```python
from build123d import *

# Parameters (mm, degrees)
BOSS_EXTRUDE1_DEPTH = 4.7625
CUT_EXTRUDE5_DEPTH  = 591.371112999
SCALE1_SCALE_X      = 0.622
SCALE1_SCALE_Y      = 0.625
SCALE1_SCALE_Z      = 1
CUT_EXTRUDE8_DEPTH  = 422.073439333
FILLET1_R           = 10.16
CUT_EXTRUDE9_DEPTH  = 422.073439333
BOSS_EXTRUDE2_DEPTH = 4.7625
CUT_EXTRUDE10_DEPTH = 422.073439333
CUT_EXTRUDE11_DEPTH = 422.073439333
SKETCH16_W          = 50.8
SKETCH16_H          = 6.35
BOSS_EXTRUDE3_DEPTH = 4.7625
CUT_EXTRUDE12_START = -4.7625
CUT_EXTRUDE12_DEPTH = 4.7625
CUT_EXTRUDE13_DEPTH = 421.232758824


# Read off the part's stored shape, not the designer's step: Cut-Extrude12
with BuildPart() as part:
    # Sketch3 → Boss-Extrude1 (new body)
    with BuildSketch(Plane.XY):
        Polygon((312.000738686, 65.991135768), (166.792028218, 317.5), (-166.792028218, 317.5), (-312.000738686, 65.991135768), (-276.650369343, 4.7625), (276.650369343, 4.7625), align=None)
        Polygon((-166.792028218, 317.5), (166.792028218, 317.5), (60.750369343, 501.169540891), (-60.750369343, 501.169540891), align=None)
    extrude(amount=BOSS_EXTRUDE1_DEPTH)

    # Sketch7 → Cut-Extrude5 (cut, through all)
    with BuildSketch(Plane.XY.offset(4.7625)):
        with BuildLine():
            Line((-147.068010972, 237.363), (147.068010972, 237.363))
            ThreePointArc((147.068010972, 237.363), (158.0665336, 243.713), (158.0665336, 256.413))
            Line((158.0665336, 256.413), (49.751846715, 444.019540891))
            ThreePointArc((49.751846715, 444.019540891), (45.103324087, 448.668063519), (38.753324087, 450.369540891))
            Line((38.753324087, 450.369540891), (-38.753324087, 450.369540891))
            ThreePointArc((-38.753324087, 450.369540891), (-45.103324087, 448.668063519), (-49.751846715, 444.019540891))
            Line((-49.751846715, 444.019540891), (-158.0665336, 256.413))
            ThreePointArc((-158.0665336, 256.413), (-158.0665336, 243.713), (-147.068010972, 237.363))
        make_face()
    extrude(amount=-CUT_EXTRUDE5_DEPTH, mode=Mode.SUBTRACT)


with BuildPart() as part_1:
    # Scale1: scaled about (0, 161.134641619, 2.38125)
    add(part.part.scale((SCALE1_SCALE_X, SCALE1_SCALE_Y, SCALE1_SCALE_Z), about=(0, 161.134641619, 2.38125)))

    # Sketch11 → Cut-Extrude8 (cut, through all)
    with BuildSketch(Plane.XY.offset(4.7625)):
        Polygon((25.4, 183.377365607), (25.4, 88.802053107), (172.163821071, 88.802053107), (117.822833735, 183.377365607), align=None)
        Polygon((-117.822833735, 183.377365607), (-25.4, 183.377365607), (-25.4, 88.802053107), (-172.163821071, 88.802053107), align=None)
    extrude(amount=-CUT_EXTRUDE8_DEPTH, mode=Mode.SUBTRACT)

    # Fillet1
    fillet1_edges = [part_1.edges().sort_by_distance(p)[0] for p in [
        (-172.163821071, 88.802053107, 2.38125),
        (-117.822833735, 183.377365607, 2.38125),
        (-25.4, 183.377365607, 2.38125),
        (-25.4, 88.802053107, 2.38125),
        (117.822833735, 183.377365607, 2.38125),
        (172.163821071, 88.802053107, 2.38125),
        (25.4, 88.802053107, 2.38125),
        (25.4, 183.377365607, 2.38125),
    ]]
    fillet(fillet1_edges, radius=FILLET1_R)

    # Sketch12 → Cut-Extrude9 (cut, through all)
    with BuildSketch(Plane.XY.offset(4.7625)):
        Polygon((141.549539127, 193.067167281), (156.734576332, 166.639056393), (153.981648115, 165.057281684), (138.796610909, 191.485392572), align=None)
        Polygon((101.309190532, 263.101661132), (98.556262314, 261.519886423), (127.660916958, 210.866007222), (130.413845176, 212.447781931), align=None)
        Polygon((-153.981648115, 165.057281684), (-138.796610909, 191.485392572), (-141.549539127, 193.067167281), (-156.734576332, 166.639056393), align=None)
        Polygon((-127.660916958, 210.866007222), (-130.413845176, 212.447781931), (-101.309190532, 263.101661132), (-98.556262314, 261.519886423), align=None)
    extrude(amount=-CUT_EXTRUDE9_DEPTH, mode=Mode.SUBTRACT)

    # Sketch13 → Boss-Extrude2 (add)
    with BuildSketch(Plane.XY.offset(4.7625)):
        Polygon((130.413845176, 212.447781931), (141.549539127, 193.067167281), (148.526307077, 197.075871548), (137.390613126, 216.456486199), align=None)
        Polygon((-148.526307077, 197.075871548), (-137.390613126, 216.456486199), (-130.413845176, 212.447781931), (-141.549539127, 193.067167281), align=None)
    extrude(amount=-BOSS_EXTRUDE2_DEPTH)

    # Sketch14 → Cut-Extrude10 (cut, through all)
    with BuildSketch(Plane.XY.offset(4.7625)):
        Polygon((172.076529731, 63.402053107), (173.900818018, 66.577053107), (121.276529731, 66.577053107), (121.276529731, 63.402053107), align=None)
        Polygon((-121.276529731, 66.577053107), (-121.276529731, 63.402053107), (-172.076529731, 63.402053107), (-173.900818018, 66.577053107), align=None)
    extrude(amount=-CUT_EXTRUDE10_DEPTH, mode=Mode.SUBTRACT)

    # Sketch15 → Cut-Extrude11 (cut, through all)
    with BuildSketch(Plane.XY.offset(4.7625)):
        Polygon((194.064459463, 101.669950462), (192.233568098, 104.85644249), (184.98443241, 92.240012302), (187.737360627, 90.658237593), align=None)
        Polygon((173.900818018, 66.577053107), (180.227916854, 77.588765977), (177.474988636, 79.170540686), (170.239035289, 66.577053107), align=None)
        Polygon((-177.474988636, 79.170540686), (-170.239035289, 66.577053107), (-173.900818018, 66.577053107), (-180.227916854, 77.588765977), align=None)
        Polygon((-187.737360627, 90.658237593), (-184.98443241, 92.240012302), (-192.233568098, 104.85644249), (-194.064459463, 101.669950462), align=None)
    extrude(amount=-CUT_EXTRUDE11_DEPTH, mode=Mode.SUBTRACT)

    # Sketch16 → Boss-Extrude3 (add)
    with BuildSketch(Plane.XY.offset(4.7625)):
        with Locations((0, 208.777365607)):
            Rectangle(SKETCH16_W, SKETCH16_H)
    extrude(amount=-BOSS_EXTRUDE3_DEPTH)

    # Cut-Extrude12 outline → Cut-Extrude12 (cut)
    with BuildSketch(Plane.XY.offset(4.7625).offset(CUT_EXTRUDE12_START)):
        Polygon((-160.03407886, 73.810353985), (-169.67848003, 77.005839249), (-172.075093978, 69.772538371), (-170.239035289, 66.577053107), (-162.430692808, 66.577053107), align=None)
    cut_extrude12 = extrude(amount=CUT_EXTRUDE12_DEPTH, mode=Mode.SUBTRACT)

    # Mirror1: Cut-Extrude12 across plane
    add(cut_extrude12.mirror(Plane(origin=(0, 0, 0), x_dir=(0, 0, 1), z_dir=(1, 0, 0))), mode=Mode.SUBTRACT)

    # Sketch18 → Cut-Extrude13 (cut, through all)
    with BuildSketch(Plane.XY.offset(4.7625)):
        Polygon((-37.786729731, 373.656453664), (37.786729731, 373.656453664), (112.762236491, 243.168725538), (-113.438180507, 243.559444472), align=None)
    extrude(amount=-CUT_EXTRUDE13_DEPTH, mode=Mode.SUBTRACT)


solid = part_1.part
```
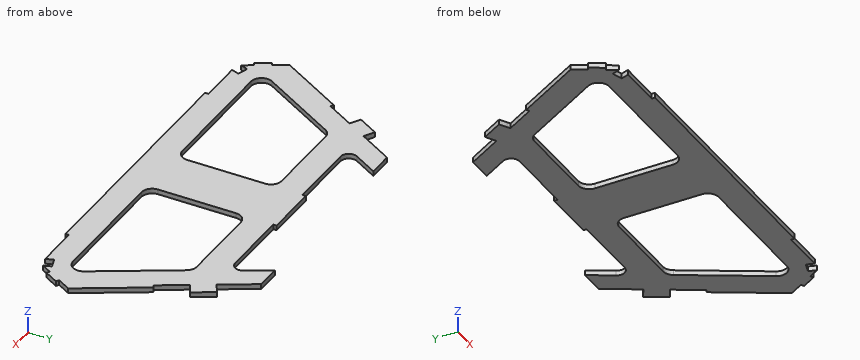
Geometry: final body of the model. Coordinates: model frame, mm. Round coordinates to 2 decimals unless told otherwise and drop trailing zeros. Order: outer loops, then holes, each group sorted by start corner. A loop starts at its lowest first (then second) coordinate and runs counter-clockwise, first axis right, second up. Notation, with made-up numbers: M -35.5,10 L -12.5,10 A18 ccw -12.5,21 Z; hole C -26.5,-16.75 d4. An arc over 180 degrees is marked long. Use one line per item in the form item = value. Start each with the question number.
Q1. Cut plane A-A (z = 1.2). Count the separate pieces of the cut face and the enclosed holes in it, and give its area (3 significant figures).
Q2. Cut plane C-C (y = 187.5). Return loops of the section in (x, z), and give its area (3 significant figures).
Q3. Pin query (flat end, axial travel): pin 1 Ø1.5 at (x, z) = (27, 1) entering from +Y; pin 2 Ø1 at (y, z) = (91, 0.5) entering from -X; pin 3 Ø2.5 at (y, z) = (144, 2.5) entering from +X. Return the tip coordinate at first contact, or that it passes through.
Q4. Material intervals for line 1 (X direction, y = 112.5, z = 3.85); line 2 (X direction, y = 214, z = 3.55); line 3 (X direction, y = 108, z = 0.6), sorted ascending. Write a range as [from, to].
Geometry results:
q1.separate_pieces = 1
q1.enclosed_holes = 2
q1.area = 28,000 mm^2
q2.outline = M -141.09,0 L 141.09,0 L 141.09,4.76 L -141.09,4.76 Z
q2.area = 1,340 mm^2
q3.pin_1 = 208.78
q3.pin_2 = -187.74
q3.pin_3 = 170.46
q4.line_1 = [-187.84, -158.55], [-25.4, 25.4], [158.55, 187.84]
q4.line_2 = [-138.8, -133.12], [-125.86, -98.9], [98.9, 125.86], [133.12, 138.8]
q4.line_3 = [-190.43, -161.13], [-25.4, 25.4], [161.13, 190.43]
